```python
from build123d import *

# Parameters (mm, degrees)
PAD041_DEPTH    = 1.2
SKETCH044_R     = 1.5
POCKET001_DEPTH = 5
SKETCH046_R     = 3
POCKET003_DEPTH = 5


with BuildPart() as part:
    # Sketch042 → Pad041 (new body)
    with BuildSketch(Plane.XY):
        with BuildLine():
            Line((-34.999999, 27), (35.000001, 27))
            ThreePointArc((38.999841, 23.000159), (37.828268, 25.828427), (35.000001, 27))
            Line((38.999841, 23.000159), (38.999841, 4.000159))
            ThreePointArc((35, 0), (37.828381, 1.171685), (38.999841, 4.000159))
            Line((35, 0), (-35, 0))
            ThreePointArc((-39.000159, 4.000159), (-37.828586, 1.171573), (-35, 0))
            Line((-39.000159, 23.00016), (-39.000159, 4.000159))
            ThreePointArc((-34.999999, 27), (-37.828473, 25.82854), (-39.000159, 23.00016))
        make_face()
    extrude(amount=PAD041_DEPTH)

    # Sketch044 (on Face10 of Pad041) → Pocket001 (cut)
    with BuildSketch(Plane.XY.offset(1.2)):
        with Locations((-35, 23)):
            Circle(SKETCH044_R)
        with Locations((35, 23)):
            Circle(SKETCH044_R)
        with Locations((35, 4)):
            Circle(SKETCH044_R)
        with Locations((-35, 4)):
            Circle(SKETCH044_R)
    extrude(amount=-POCKET001_DEPTH, mode=Mode.SUBTRACT)

    # Sketch046 (on Face5 of Pocket001) → Pocket003 (cut)
    with BuildSketch(Plane.XY.offset(1.2)):
        with Locations((-26, 13.5)):
            Circle(SKETCH046_R)
    extrude(amount=-POCKET003_DEPTH, mode=Mode.SUBTRACT)


with BuildPart() as part_1:
    # Body015 placement: moved
    add(part.part.moved(Location((0, 0, 120))))


solid = part_1.part
```
CAD build for the part. Positions are in the model's coordinates, mm. Round coordinates to 2 decimals unless told otherwise and drop trailing zeros. Write each loop counter-clockwise with the first axis right and the second up, starting at its lowest first coordinate (ties: lowest second). Pieces come first, ordered by that corner, then holes.
Item 1: Drill centre lines: L1, parallel to X at y = 3.25, z = 120.3; L2, parallel to X at y = 13.25, z = 121.05; L3, parallel to X at y = 5, z = 120.1. Where is each one in solid material? Low to high.
Filled in:
L1: x = -38.93 to -36.3, -33.7 to 33.7, 36.3 to 38.93
L2: x = -39 to -28.99, -23.01 to 39
L3: x = -39 to -36.12, -33.88 to 33.88, 36.12 to 39
Item 2: Mould opens along X. For faces 1 (the cylindrical face through (33.89, 24.01, 120.61)), 2 (the cylindrical face through (-37.797, 25.859, 120.592)), 3 (the flat face through (1, 14, 120)) say: released by +X, released by -X, zero draft, split by the parting line, or undercut.
Filled in:
face 1: undercut
face 2: released by -X
face 3: zero draft
Item 3: Band-saw the part on B-B on z = 120.25. Write the cut outline in (x, y), then the cut area to 3 significant figures.
Filled in:
outline: (-39, 4) arc R4 ccw to (-35, 0) - (35, 0) arc R4 ccw to (39, 4) - (39, 23) arc R4 ccw to (35, 27) - (-35, 27) arc R4 ccw to (-39, 23) - close; hole circle Ø3 at (-35, 4); hole circle Ø3 at (-35, 23); hole circle Ø6 at (-26, 13.5); hole circle Ø3 at (35, 4); hole circle Ø3 at (35, 23)
area: 2,040 mm2
Item 4: Band-saw the part on A-A on y = 13.5. Write the cut outline in (x, z).
Filled in:
outline: (-39, 120) - (-29, 120) - (-29, 121.2) - (-39, 121.2) - close; (-23, 120) - (39, 120) - (39, 121.2) - (-23, 121.2) - close
